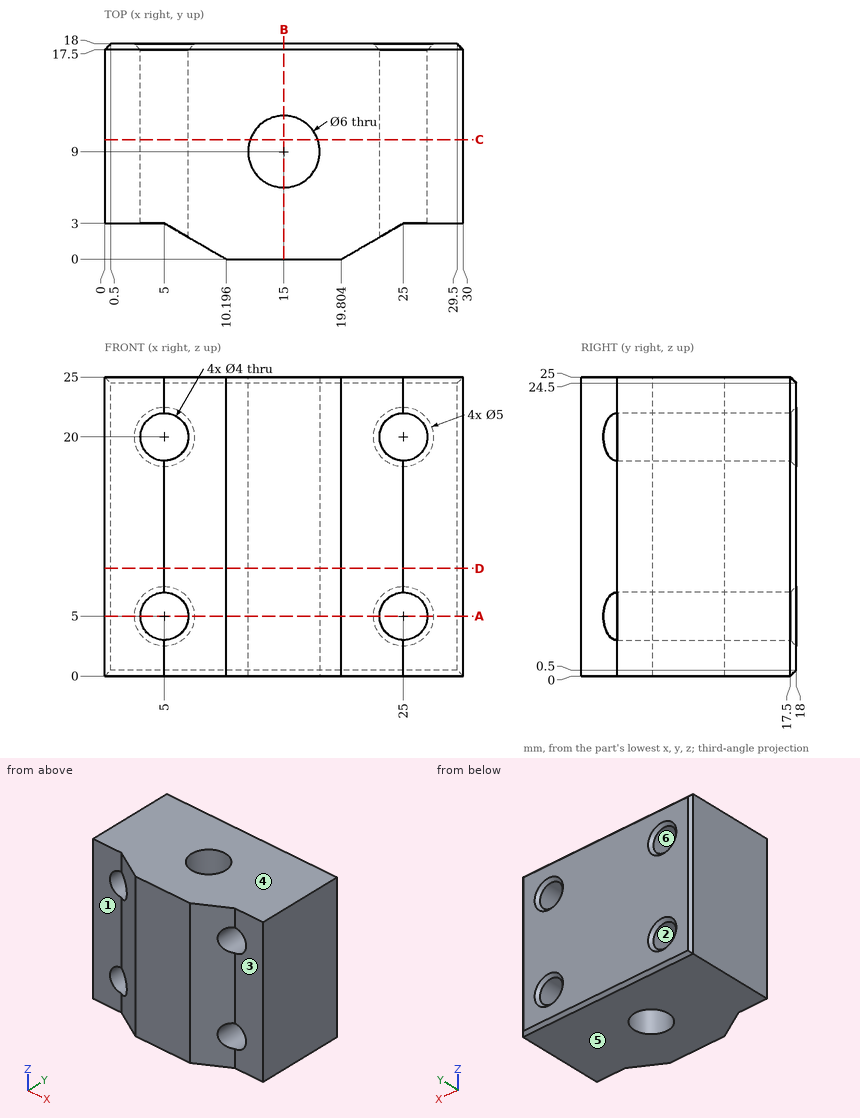
Here's the drawing with two shaded views (mm, measured from the low corner). I have some questions. A direction names the side the tool comes from. Round coordinates to 2 decimals unless told otherwise and drop trailing zeros. Loops run counter-clockwise (first coordinate to the right, second up) from the corner with the lowest first, then second, coordinate; pieces in that order, holes last. Notation, with made-up numbers: (-6, -26.5) -> (48, -26.5) arc R30 cw to (48, 3.5) -> close; hole circle Ø8 at (79, 64). An arc over 180 degrees is marked (long way). Answer as CSV lines item,"result". Start each with the question number.
1. For the marked faces 1, 2 and 3, which set-ups out of +Z, -Z, +X, -X, +Y, -Y let a thin tool reach every point of the face, with its end or its side?
2. Imagine slicing it at D-D on z = 9. Write out the boundary of the cut face in (x, y), plus the area to 3 significant figures.
3. If we mould it in two halves opening along Z, with no side actions, what happens to the marked faces 4, 5 and 6? For each: pulls with the +Z half, pulls with the -Z half, needs draft (parallel to the pull), parting line crosses it, or undercut.
4. I'm going to push flat-ended pins straight in: P1, Ø2.5, axis at x = 5, z = 5, coming from the +Y side; P2, Ø4.5, axis at x = 5, z = 20, coming from the +Y side; P3, Ø2.5, axis at x = 28.5, z = 10, coming from the -Y side; P4, Ø4.5, axis at x = 25, z = 5, coming from the -Y side. Where does each tip first touch, or does it pass through?
5. Imagine slicing it at B-B on x = 15. Write out the boundary of the cut face in (y, z), plus the area to 3 significant figures.
6. Imagine slicing it at A-A on z = 5. Write out the boundary of the cut face in (x, y) (1 decimal), plus the area to 3 significant figures.
7. I need wall thicknesses on probe 1 along Z at (x, y) = (25, 10); probe 2 along Z at (x, y) = (25.5, 3.5); probe 3 along X at (y, z) = (9.5, 20). Which ranges of each line are inside material? Lowest first, please. Write a range as from..to.
8. Imagine slicing it at C-C on y = 10. Write out the boundary of the cut face in (x, z).
Solution:
1,face 1,"+Z, -Z, -X, -Y"
1,face 2,"+Y, -Y"
1,face 3,"+Z, -Z, +X, -Y"
2,outline,"(0, 3) -> (5, 3) -> (10.2, 0) -> (19.8, 0) -> (25, 3) -> (30, 3) -> (30, 17.5) -> (29.5, 18) -> (0.5, 18) -> (0, 17.5) -> close; hole circle Ø6 at (15, 9)"
2,area,"466 mm²"
3,face 4,"pulls with the +Z half"
3,face 5,"pulls with the -Z half"
3,face 6,"undercut"
4,P1,"through"
4,P2,"y = 17.75"
4,P3,"y = 3"
4,P4,"y = 1.7"
5,outline,"(0, 0) -> (6, 0) -> (6, 25) -> (0, 25) -> close; (12, 0) -> (17.5, 0) -> (18, 0.5) -> (18, 24.5) -> (17.5, 25) -> (12, 25) -> close"
5,area,"300 mm²"
6,outline,"(0, 3) -> (3, 3) -> (3, 17.5) -> (2.5, 18) -> (0.5, 18) -> (0, 17.5) -> close; (7, 1.8) -> (10.2, 0) -> (19.8, 0) -> (23, 1.8) -> (23, 17.5) -> (22.5, 18) -> (7.5, 18) -> (7, 17.5) -> close; (27, 3) -> (30, 3) -> (30, 17.5) -> (29.5, 18) -> (27.5, 18) -> (27, 17.5) -> close; hole circle Ø6 at (15, 9)"
6,area,"343 mm²"
7,probe 1,"0..3, 7..18, 22..25"
7,probe 2,"0..3.06, 6.94..18.06, 21.94..25"
7,probe 3,"0..3, 7..12.04, 17.96..23, 27..30"
8,outline,"(0, 0) -> (12.17, 0) -> (12.17, 25) -> (0, 25) -> close; (17.83, 0) -> (30, 0) -> (30, 25) -> (17.83, 25) -> close; hole circle Ø4 at (5, 5); hole circle Ø4 at (5, 20); hole circle Ø4 at (25, 5); hole circle Ø4 at (25, 20)"
